from build123d import *

# Parameters (mm, degrees)
F0_R     = 1.5875
F1_DEPTH = 3.048


with BuildPart() as f1:
    # F0 (on Front) → F1 (new body)
    with BuildSketch(Plane.XZ):
        with BuildLine():
            ThreePointArc((-9.525, 50.8), (0, 41.275), (9.525, 50.8))
            ThreePointArc((9.525, 50.8), (0, 60.325), (-9.525, 50.8))
        make_face()
        with Locations((0, 50.8)):
            Circle(F0_R, mode=Mode.SUBTRACT)
        with BuildLine():
            Line((15.386538, 3.907692), (9.525, 50.8))
            ThreePointArc((9.525, 50.8), (0, 41.275), (-9.525, 50.8))
            Line((-9.525, 50.8), (-15.747457, 2.00829))
            ThreePointArc((-15.747457, 2.00829), (-0.966694, 15.84554), (15.386538, 3.907692))
        make_face()
        with Locations((-3.175, 36.5252)):
            Circle(F0_R, mode=Mode.SUBTRACT)
        with BuildLine():
            Line((15.875, 0), (15.386538, 3.907692))
            ThreePointArc((15.386538, 3.907692), (-0.966694, 15.84554), (-15.747457, 2.00829))
            ThreePointArc((-15.747457, 2.00829), (-2.57762, -15.664338), (15.560644, -3.143564))
            Line((15.560644, -3.143564), (15.875, 0))
        make_face()
        Circle(F0_R, mode=Mode.SUBTRACT)
        with BuildLine():
            ThreePointArc((15.560644, -3.143564), (-2.57762, -15.664338), (-15.747457, 2.00829))
            Line((-15.747457, 2.00829), (-16.003576, 0))
            Line((-16.003576, 0), (-9.525, -63.5))
            ThreePointArc((-9.525, -63.5), (0, -53.975), (9.525, -63.5))
            ThreePointArc((9.525, -63.5), (6.970557, -69.991299), (0.677344, -73.000886))
            Line((0.677344, -73.000886), (44.732405, -71.432475))
            ThreePointArc((44.732405, -71.432475), (36.513756, -63.641225), (44.45, -55.5625))
            Line((44.45, -55.5625), (18.910573, -54.650378))
            ThreePointArc((18.910573, -54.650378), (13.205355, -51.933808), (11.283583, -45.914169))
            Line((11.283583, -45.914169), (15.560644, -3.143564))
        make_face()
        with BuildLine():
            ThreePointArc((52.3875, -63.5), (50.06266, -57.88734), (44.45, -55.5625))
            ThreePointArc((44.45, -55.5625), (36.513756, -63.641225), (44.732405, -71.432475))
            ThreePointArc((44.732405, -71.432475), (50.161633, -69.01191), (52.3875, -63.5))
        make_face()
        with Locations((44.45, -63.5)):
            Circle(F0_R, mode=Mode.SUBTRACT)
        with BuildLine():
            ThreePointArc((9.525, -63.5), (0, -53.975), (-9.525, -63.5))
            ThreePointArc((-9.525, -63.5), (-6.735192, -70.235192), (0, -73.025))
            Line((0, -73.025), (0.677344, -73.000886))
            ThreePointArc((0.677344, -73.000886), (6.970557, -69.991299), (9.525, -63.5))
        make_face()
        with Locations((0, -63.5)):
            Circle(F0_R, mode=Mode.SUBTRACT)
    extrude(amount=F1_DEPTH)


solid = f1.part
Could you check a few things on this model? Use its own coordinates, in mm. Give positions to 0.01 mm unless a question says otherwise; leave off trailing zeros. Write each loop counter-clockwise with the first axis right and the second up, starting at its lowest first coordinate (ties: lowest second). Pieces come first, ordered by that corner, then holes. Notation, with made-up numbers: (71, -11.5) -> (88, -11.5) arc R9 ccw to (88, 4.5) -> close; hole circle Ø3 at (-18, 15.5). An arc over 180 degrees is marked (long way). Write each question's results on one line, items separated by ' | '. Start each with the question number.
Q1. We'd pull the mould along X, two halves only. Please class faces 1 (the face through (-6.81, -1.5, -70.16)), 2 (the face through (13.266, -1.503, -52.002)), 3 (the face through (0.85, -1.5, 52.14)), 4 (the face through (-0.34, -1.5, -1.55)): +X half, -X half, draft (parallel to the pull), parting line (faces both ways), or undercut.
Q2. Suppose I cut it at B-B, the plane z = -31. List the corners of the cut face in (x, y) for me (3 decimals).
Q3. Suppose I cut it at C-C, the plane x = 33. List the corners of the cut face in (y, z) for me, and give its area (3 significant figures).
Q4. Suppose I cut it at A-A, the plane y = -1.75. State how many separate pieces and enclosed holes the cut face has, and give its area (3 significant figures).
Q5. I need wall thicknesses on probe 1 along Z at (x, y) = (1, -2.65); probe 2 along Z at (x, y) = (-2, -2.2); probe 3 along Z at (x, y) = (-4, -1.7). Which ranges of each line are inside material? Lowest first, please.
Outcome:
1) face 1: -X half | face 2: +X half | face 3: undercut | face 4: undercut
2) outline: (-12.841, -3.048) -> (12.775, -3.048) -> (12.775, 0) -> (-12.841, 0) -> close
3) outline: (-3.05, -71.85) -> (0, -71.85) -> (0, -55.15) -> (-3.05, -55.15) -> close | area: 50.9 mm2
4) separate pieces: 1 | enclosed holes: 5 | area: 3,880 mm2
5) probe 1: -72.99 to -64.73, -62.27 to -1.23, 1.23 to 49.57, 52.03 to 60.27 | probe 2: -72.81 to 35.46, 37.59 to 60.11 | probe 3: -72.14 to 35.17, 37.88 to 59.44
